Part model, mm, in its own coordinate system. Round coordinates to 2 decimals unless told otherwise and drop trailing zeros. Order: outer loops, then holes, each group sorted by start corner. A loop starts at its lowest first (then second) coordinate and runs counter-clockwise, first axis right, second up. Notation, with made-up numbers: (-1.5, 55) - (15.5, 55) arc R28 ccw to (15.5, 91) - close; hole circle Ø3 at (-21.5, -24.5). An arc over 180 degrees is marked (long way). Answer as a JSON object with one key per item and string values.
```python
from build123d import *

# Parameters (mm, degrees)
SKETCH2_R      = 1.1811
EXTRUDE1_DEPTH = 1.5748
FILLET1_R      = 0.254


with BuildPart() as part:
    # Sketch2 → Extrude1 (new body)
    with BuildSketch(Plane(origin=(0, 0, 0), x_dir=(1, 0, 0), z_dir=(0, 1, 0))):
        with BuildLine():
            Line((11.389308583, -24.424451076), (10.079527634, -21.615616767))
            ThreePointArc((10.079527634, -21.615616767), (10.334109559, -18.705732054), (12.981434605, -17.471264112))
            Line((12.981434605, -17.471264112), (17.211887304, -17.841380764))
            ThreePointArc((17.211887304, -17.841380764), (0, 22.6314), (-17.211887304, -17.841380764))
            Line((-17.211887304, -17.841380764), (-12.981434605, -17.471264112))
            ThreePointArc((-12.981434605, -17.471264112), (-10.334109559, -18.705732054), (-10.079527634, -21.615616767))
            Line((-10.079527634, -21.615616767), (-11.389308583, -24.424451076))
            ThreePointArc((-11.389308583, -24.424451076), (0, 26.9494), (11.389308583, -24.424451076))
        make_face()
        with Locations((12.72685268, -20.381148825)):
            Circle(SKETCH2_R, mode=Mode.SUBTRACT)
        with Locations((-12.72685268, -20.381148825)):
            Circle(SKETCH2_R, mode=Mode.SUBTRACT)
    extrude(amount=-EXTRUDE1_DEPTH)

    # Fillet1
    fillet1_edges = [part.edges().sort_by_distance(p)[0] for p in [
        (17.211887304, -0.7874, 17.841380764),
        (-17.211887304, -0.7874, 17.841380764),
    ]]
    fillet(fillet1_edges, radius=FILLET1_R)


solid = part.part
```
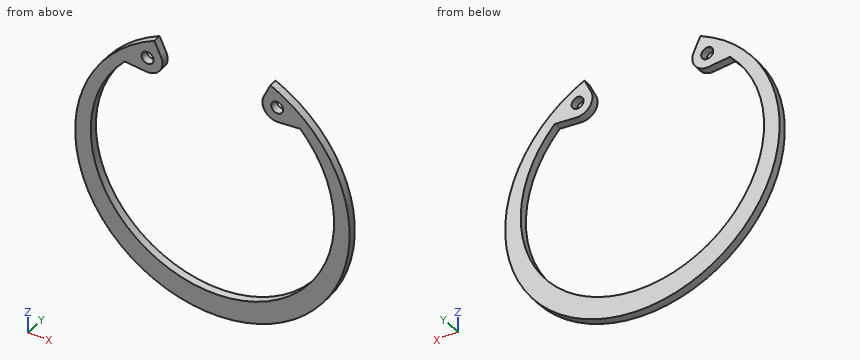
Item 1: Cut at A-A (z = 14.5). Write the cut outline in (x, y), plus the area to 3 significant figures.
Taken from the geometry:
{"outline": "(-22.72, -1.57) - (-19.9, -1.57) - (-19.9, 0) - (-22.72, 0) - close; (19.9, -1.57) - (22.72, -1.57) - (22.72, 0) - (19.9, 0) - close", "area": "8.88 mm2"}
Item 2: Probe L1, parallel to Z at x = 13, y = -0.5; L2, parallel to X at y = -1.15, z = -3.5; L3, parallel to Z at x = -19, y = -1.45. List the from-to ranges inside material, lowest first. Write a range as from..to.
Taken from the geometry:
{"L1": "-23.61..-18.79, 17.47..19.23, 21.53..23.61", "L2": "-26.72..-23.42, 23.42..26.72", "L3": "-19.11..-13.23, 15.76..19.11"}
Item 3: Cut at B-B (y = -0.75). Write the cut outline in (x, z), plus the area to 3 significant figures.
Taken from the geometry:
{"outline": "(-17.3, 17.75) arc R0.25 cw to (-17.09, 17.83) - (-12.98, 17.47) arc R2.92 ccw to (-10.08, 21.62) - (-11.39, 24.42) arc R26.95 ccw (long way) to (11.39, 24.42) - (10.08, 21.62) arc R2.92 ccw to (12.98, 17.47) - (17.09, 17.83) arc R0.25 cw to (17.3, 17.75) arc R23.9 cw (long way) to start; hole circle Ø2.36 at (-12.73, 20.38); hole circle Ø2.36 at (12.73, 20.38)", "area": "480 mm2"}
Item 4: Cut at D-D (z = 0). Write the cut outline in (x, y).
Taken from the geometry:
{"outline": "(-26.95, -1.57) - (-23.86, -1.57) - (-23.86, 0) - (-26.95, 0) - close; (23.86, -1.57) - (26.95, -1.57) - (26.95, 0) - (23.86, 0) - close"}
Item 5: Cut at C-C (x = 0). Write the cut outline in (y, z), plus the area to 3 significant figures.
Taken from the geometry:
{"outline": "(-1.57, -26.95) - (0, -26.95) - (0, -22.63) - (-1.57, -22.63) - close", "area": "6.80 mm2"}
